```python
from build123d import *

# Parameters (mm, degrees)
F0_W     = 133
F0_H     = 72
F1_DEPTH = 36
F2_W     = 10
F2_H     = 50
F3_DEPTH = 2
F5_DEPTH = 2


with BuildPart() as f1:
    # F0 (on Top) → F1 (new body)
    with BuildSketch(Plane.XY):
        Rectangle(F0_W, F0_H)
    extrude(amount=F1_DEPTH)

    # F2 (on face) → F3 (join)
    with BuildSketch(Plane(origin=(0, 0, 0), x_dir=(1, 0, 0), z_dir=(0, 0, -1))):
        with Locations((-71.5, 0)):
            Rectangle(F2_W, F2_H)
        with BuildLine():
            ThreePointArc((-69, -20), (-71.627534, -22.496745), (-73.986988, -19.745264))
            Line((-73.986988, -19.745264), (-73.986988, -12.254736))
            ThreePointArc((-73.986988, -12.254736), (-74, -12), (-73.986988, -11.745264))
            ThreePointArc((-73.986988, -11.745264), (-71.372466, -9.503255), (-69, -12))
            Line((-69, -12), (-69, -20))
        make_face(mode=Mode.SUBTRACT)
        with BuildLine():
            ThreePointArc((-73.944746, 19.477297), (-71.5, 22.5), (-69.055254, 19.477297))
            Line((-69.055254, 19.477297), (-69.055254, 12.522703))
            ThreePointArc((-69.055254, 12.522703), (-71.5, 9.5), (-73.944746, 12.522703))
            Line((-73.944746, 12.522703), (-73.944746, 19.477297))
        make_face(mode=Mode.SUBTRACT)
    extrude(amount=-F3_DEPTH)

    # F4 (on face) → F5 (join)
    with BuildSketch(Plane(origin=(0, 0, 0), x_dir=(1, 0, 0), z_dir=(0, 0, -1))):
        Polygon((66.5, 0), (66.5, -25), (76.5, -25), (76.5, 25), (66.5, 25), align=None)
        with BuildLine():
            ThreePointArc((73.944746, -19.477297), (71.5, -22.5), (69.055254, -19.477297))
            Line((69.055254, -19.477297), (69.055254, -12.522703))
            ThreePointArc((69.055254, -12.522703), (71.5, -9.5), (73.944746, -12.522703))
            Line((73.944746, -12.522703), (73.944746, -19.477297))
        make_face(mode=Mode.SUBTRACT)
        with BuildLine():
            ThreePointArc((69, 20), (71.627534, 22.496745), (73.986988, 19.745264))
            Line((73.986988, 19.745264), (73.986988, 12.254736))
            ThreePointArc((73.986988, 12.254736), (74, 12), (73.986988, 11.745264))
            ThreePointArc((73.986988, 11.745264), (71.372466, 9.503255), (69, 12))
            Line((69, 12), (69, 20))
        make_face(mode=Mode.SUBTRACT)
    extrude(amount=-F5_DEPTH)


solid = f1.part
```
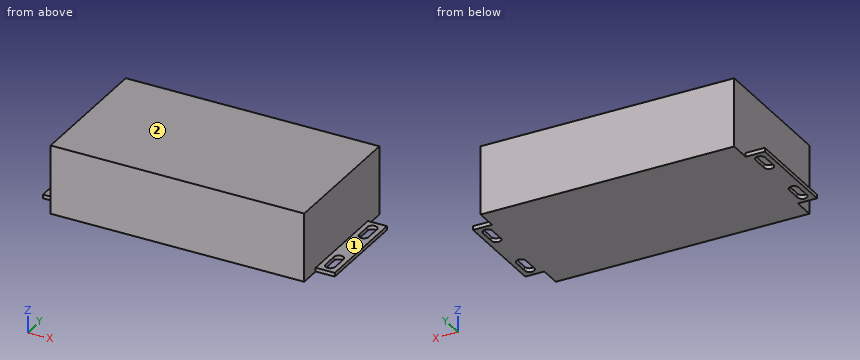
Input: part model. Units: mm. Frame: model coordinates. Face numbers are marked on the shaded views. A direction names the side the tool comes from. Round coordinates to 2 decimals unless told otherwise and drop trailing zeros. Loops run counter-clockwise (first coordinate to the right, second up) from the corner with the lowest first, then second, coordinate; pieces in that order, holes last.
1) Set-up query: the marked faces 1 and 2. Return all of +Z, -Z, +X, -X, +Y, -Y with unobstructed straight access to the full face (end or side cutting, diameter ignored); none if empty.
Ans:
face 1: +Z, +X, +Y, -Y
face 2: +Z, +X, -X, +Y, -Y
2) Section query C-C on y = 2.5. Return the cut outline in (x, z), plus the area to 3 significant figures.
Ans:
outline: (-76.5, 0) - (76.5, 0) - (76.5, 2) - (66.5, 2) - (66.5, 36) - (-66.5, 36) - (-66.5, 2) - (-76.5, 2) - close
area: 4,830 mm2
3) Section query B-B on x = 71.5. Return the cut outline in (y, z), plus the area to 3 significant figures.
Ans:
outline: (-25, 0) - (-22.5, 0) - (-22.5, 2) - (-25, 2) - close; (-9.5, 0) - (9.5, 0) - (9.5, 2) - (-9.5, 2) - close; (22.5, 0) - (25, 0) - (25, 2) - (22.5, 2) - close
area: 48.0 mm2
4) Pin query (flat end, axial travel): pin 1 (5 mm diameter, centred on x = -71, y = 7.5, fed in from +Z); pin 2 (2 mm diameter, centred on x = 74, z = 1.5, fed in from -Y); pin 3 (2 mm diameter, centred on x = -72, z = 0.5, fed in from +Y); pin 4 (6 mm diameter, centred on x = 71.5, y = 12, fed in from -Z). Return the tip coordinate at first contact, or that it passes through.
Ans:
pin 1: stops at z = 2
pin 2: stops at y = -25
pin 3: stops at y = 25
pin 4: stops at z = 0
5) Material intervals for line 1 (X direction, y = 20, z = 1.5); line 2 (Y direction, x = 71.5, z = 1.3); line 3 (Z direction, x = 68, y = 8), sorted ascending.
Ans:
line 1: x = -76.5 to -74, -69 to 69, 74 to 76.5
line 2: y = -25 to -22.5, -9.5 to 9.5, 22.5 to 25
line 3: z = 0 to 2
6) Section query D-D on z = 24.5. Return the cut outline in (x, y), plus the area to 3 significant figures.
Ans:
outline: (-66.5, -36) - (66.5, -36) - (66.5, 36) - (-66.5, 36) - close
area: 9,580 mm2
7) Section query A-A on y = -15. Return the cut outline in (x, z), plus the area to 3 significant figures.
Ans:
outline: (-76.5, 0) - (-73.94, 0) - (-73.94, 2) - (-76.5, 2) - close; (-69.06, 0) - (69, 0) - (69, 2) - (66.5, 2) - (66.5, 36) - (-66.5, 36) - (-66.5, 2) - (-69.06, 2) - close; (73.99, 0) - (76.5, 0) - (76.5, 2) - (73.99, 2) - close
area: 4,810 mm2
